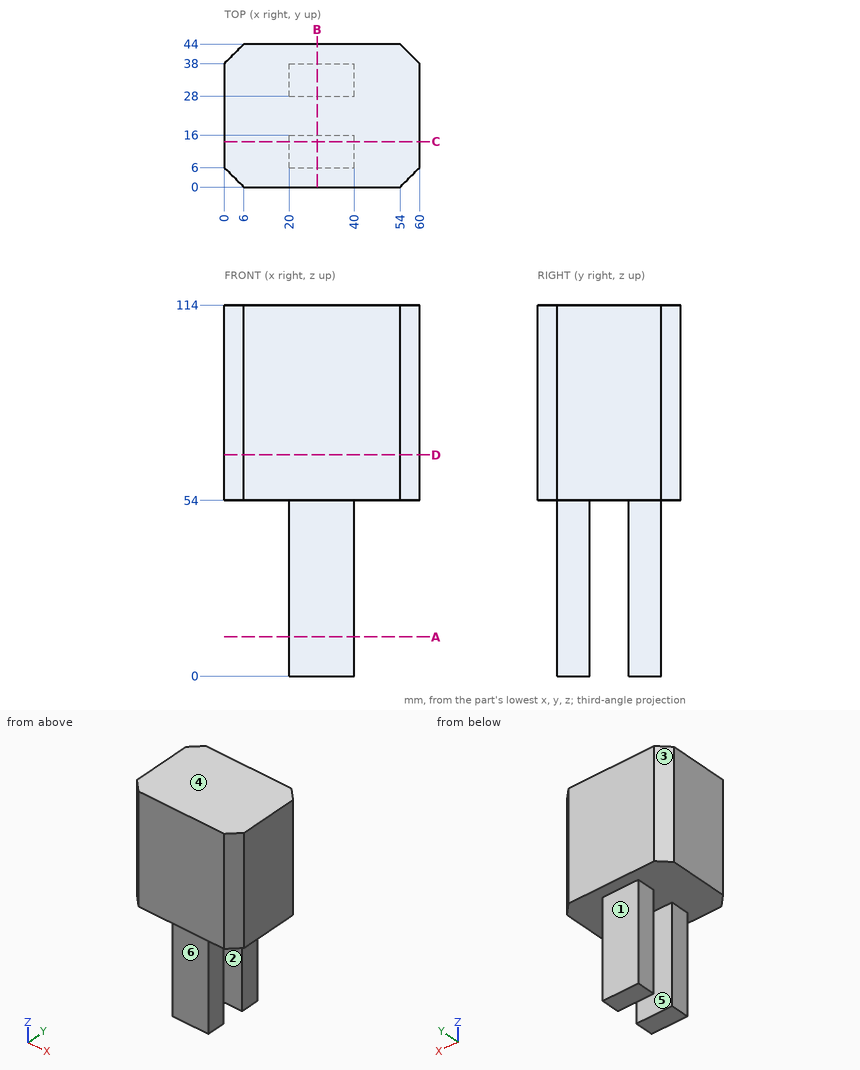
Part print with two shaded views. Sizes in mm from the minimum x, y, z corner. A direction names the side the tool comes from. Round coordinates to 2 decimals unless told otherwise and drop trailing zeros. Order: outer loops, then holes, each group sorted by start corner. A loop starts at its lowest first (then second) coordinate and runs counter-clockwise, first axis right, second up. Notation, with made-up numbers: M -11.5,-16.5 L 6.5,-16.5 A24 cw 6.5,6.5 Z; hole C 70,-13.5 d1. An arc over 180 degrees is marked long. Put each result on its own line as item: value. Start each with the question number.
1. Drill centre lines: probe 1 along Y at (x, z) = (35.5, 18); probe 2 along Z at (x, y) = (53.5, 23); probe 3 along X at (y, z) = (31.5, 17). Where is each one in solid material? Low to high. Write a range as [from, to].
2. Drop flat-ended pins along their axis: pin 1 (1 mm diameter, centred on x = 22.5, z = 37, fed in from -Y); pin 2 (2 mm diameter, centred on y = 17.5, z = 36.5, fed in from -X); pin 3 (8 mm diameter, centred on y = 33, z = 24, fed in from +X); pin 4 (3 mm diameter, centred on y = 13, z = 16.5, fed in from -X). Give the stop position or say it passes through.
3. Tool access for the marked faces 1, 2 and 3: list every direction of +Z, -Z, +X, -X, +Y, -Y with a clear straight run to the whole face (end or side of a thin tool).
4. Slice it at D-D on z = 68. List the corners of the cut face in (x, y), then the cut area to 3 significant figures.
5. Slice it at B-B on x = 28.5. List the corners of the cut face in (y, z).
6. Two-plate mould, pull along Y, no slides. Class the marked faces 4, 5 and 6: +Y half, -Y half, draft (parallel to the pull), parting line (faces both ways), or undercut.
7. Slice it at C-C on y = 14. List the corners of the cut face in (x, z).
8. Slice it at A-A on z = 12. List the corners of the cut face in (x, y).
Findings:
1. probe 1: [6, 16], [28, 38]
1. probe 2: [54, 114]
1. probe 3: [20, 40]
2. pin 1: y = 6
2. pin 2: through
2. pin 3: x = 40
2. pin 4: x = 20
3. face 1: -Z, +X, -X, +Y
3. face 2: -Z, +X, -X
3. face 3: +Z, -Z, -X, +Y
4. outline: M 0,6 L 6,0 L 54,0 L 60,6 L 60,38 L 54,44 L 6,44 L 0,38 Z
4. area: 2,570 mm2
5. outline: M 0,54 L 6,54 L 6,0 L 16,0 L 16,54 L 28,54 L 28,0 L 38,0 L 38,54 L 44,54 L 44,114 L 0,114 Z
6. face 4: draft
6. face 5: undercut
6. face 6: -Y half
7. outline: M 0,54 L 20,54 L 20,0 L 40,0 L 40,54 L 60,54 L 60,114 L 0,114 Z
8. outline: M 20,6 L 40,6 L 40,16 L 20,16 Z; M 20,28 L 40,28 L 40,38 L 20,38 Z
